```python
from build123d import *

# Parameters (mm, degrees)
F0_R            = 37.5
F1_DEPTH        = 20
F2_R            = 2
F3_DEPTH        = 20.001
F3_COPIES_COUNT = 6
F5_DEPTH        = 3.25
F5_COPIES_COUNT = 6
F6_R            = 7.5
F7_DEPTH        = 4.15
F8_W            = 7
F8_H            = 7
F9_DEPTH        = 4
F10_W           = 47
F10_H           = 3.18
F11_DEPTH       = 8.15
F12_R           = 3.25
F13_DEPTH       = 11.851


# Not quite as in the source:
# - a pattern or mirror of a feature is missing from the dataset's text; its kind, count and spacing are read off the source's solid


with BuildPart() as f1:
    # F0 (on Front) → F1 (new body)
    with BuildSketch(Plane.XZ):
        Circle(F0_R)
    extrude(amount=F1_DEPTH)

    # F2 (on Front) → F3 (cut, through all)
    with BuildSketch(Plane.XZ):
        with Locations((0, 30)):
            Circle(F2_R)
    f3 = extrude(amount=F3_DEPTH, mode=Mode.SUBTRACT)

    # F3_copies: F3 ×6 about axis
    f3_copies_axis = Axis((0, 0, 0), (0, 1, 0))
    for i in range(1, F3_COPIES_COUNT):
        add(f3.rotate(f3_copies_axis, i * 360 / F3_COPIES_COUNT), mode=Mode.SUBTRACT)

    # F4 (on face) → F5 (cut)
    with BuildSketch(Plane.XZ.offset(20)):
        Polygon((2.3749, 34.1134474629), (-2.3749, 34.1134474629), (-4.7498, 30), (-2.3749, 25.8865525371), (2.3749, 25.8865525371), (4.7498, 30), align=None)
    f5 = extrude(amount=-F5_DEPTH, mode=Mode.SUBTRACT)

    # F5_copies: F5 ×6 about axis
    f5_copies_axis = Axis((0, 0, 0), (0, 1, 0))
    for i in range(1, F5_COPIES_COUNT):
        add(f5.rotate(f5_copies_axis, i * 360 / F5_COPIES_COUNT), mode=Mode.SUBTRACT)

    # F6 (on face) → F7 (cut)
    with BuildSketch(Plane(origin=(0, 0, 0), x_dir=(-1, 0, 0), z_dir=(0, 1, 0))):
        Circle(F6_R)
    extrude(amount=-F7_DEPTH, mode=Mode.SUBTRACT)

    # F8 (on face) → F9 (cut)
    with BuildSketch(Plane(origin=(0, -4.15, 0), x_dir=(-1, 0, 0), z_dir=(0, 1, 0))):
        Rectangle(F8_W, F8_H)
    extrude(amount=-F9_DEPTH, mode=Mode.SUBTRACT)

    # F10 (on face) → F11 (cut, through all)
    with BuildSketch(Plane(origin=(0, 0, 0), x_dir=(-1, 0, 0), z_dir=(0, 1, 0))):
        Rectangle(F10_W, F10_H)
    extrude(amount=-F11_DEPTH, mode=Mode.SUBTRACT)

    # F12 (on face) → F13 (cut, through all)
    with BuildSketch(Plane(origin=(0, -8.15, 0), x_dir=(-1, 0, 0), z_dir=(0, 1, 0))):
        Circle(F12_R)
    extrude(amount=-F13_DEPTH, mode=Mode.SUBTRACT)


solid = f1.part
```
Geometry: final body of the model. Coordinates: model frame, mm. A direction names the side the tool comes from. Coordinates: 2 decimals unless noted, no trailing zeros. Loops run counter-clockwise (first coordinate to the right, second up) from the corner with the lowest first, then second, coordinate; pieces in that order, holes last. Notation, with made-up numbers: (61, 39.5) -> (80, 39.5) arc R33 cw to (80, 76.5) -> close; hole circle Ø5 at (-6, 67). An arc over 180 degrees is marked (long way). Use a Markdown table: item, result. Add a question column.
(1) Section query B-B, the plane y = -5.25. Return loops of the section in (x, z).
(2) Line query: line 1 along Z through (x, y) = (0, -12.5); line 2 along Z through (x, y) = (-26, -1); line 3 along Z through (x, y) = (21.5, -13.75). Output: solid intervals per line, ascending.
(3) Section query A-A, the plane z = 0. Return loops of the section in (x, y), plus the area to 3 significant figures.
(4) Section query C-C, the plane x = -19. Return loops of the section in (y, z), plus the area to 3 significant figures.
(5) Section query D-D, the plane y = -13. Return loops of the section in (x, z).
(6) Pin query (flat end, axial travel): pin 1 Ø1.6 at (x, y) = (0, -19) entering from -Z; pin 2 Ø2.5 at (x, z) = (0, 30) entering from -Y; pin 3 Ø0.6 at (y, z) = (-5.5, 2) entering from +X; pin 4 Ø4 at (x, y) = (-11.5, -3) entering from +Z. Return the tip coordinate at first contact, or that it passes through.
(7) Access query for faces 1 (the flat face through (-13, -4, 1.59)), 2 (the flat face through (26, -18, 19.113)), 3 (the cylindrical face through (-24.073, -8.258, -14.399)). Directions: +Z, -Z, +X, -X, +Y, -Y. A direction counts if a zero-diameter tool reaches every point of the face in a straight line with its end or side. Return the directions, or none.
Answer:
| question | item | result |
|---|---|---|
| 1 | outline | circle Ø75 at (0, 0); hole circle Ø4 at (-25.98, -15); hole circle Ø4 at (-25.98, 15); hole (-23.5, -1.59) -> (-3.5, -1.59) -> (-3.5, -3.5) -> (3.5, -3.5) -> (3.5, -1.59) -> (23.5, -1.59) -> (23.5, 1.59) -> (3.5, 1.59) -> (3.5, 3.5) -> (-3.5, 3.5) -> (-3.5, 1.59) -> (-23.5, 1.59) -> close; hole circle Ø4 at (0, -30); hole circle Ø4 at (0, 30); hole circle Ø4 at (25.98, -15); hole circle Ø4 at (25.98, 15) |
| 2 | line 1 | z = -37.5 to -32, -28 to -3.25, 3.25 to 28, 32 to 37.5 |
| 2 | line 2 | z = -27.02 to -17, -13 to 13, 17 to 27.02 |
| 2 | line 3 | z = -30.72 to 30.72 |
| 3 | outline | (-37.5, -20) -> (-3.25, -20) -> (-3.25, -8.15) -> (-23.5, -8.15) -> (-23.5, 0) -> (-37.5, 0) -> close; (3.25, -20) -> (37.5, -20) -> (37.5, 0) -> (23.5, 0) -> (23.5, -8.15) -> (3.25, -8.15) -> close |
| 3 | area | 1,040 mm^2 |
| 4 | outline | (-20, -32.33) -> (0, -32.33) -> (0, -1.59) -> (-8.15, -1.59) -> (-8.15, 1.59) -> (0, 1.59) -> (0, 32.33) -> (-20, 32.33) -> close |
| 4 | area | 1,270 mm^2 |
| 5 | outline | circle Ø75 at (0, 0); hole circle Ø4 at (-25.98, -15); hole circle Ø4 at (-25.98, 15); hole circle Ø6.5 at (0, 0); hole circle Ø4 at (0, -30); hole circle Ø4 at (0, 30); hole circle Ø4 at (25.98, -15); hole circle Ø4 at (25.98, 15) |
| 6 | pin 1 | stops at z = -37.5 |
| 6 | pin 2 | passes through |
| 6 | pin 3 | stops at x = 37.46 |
| 6 | pin 4 | stops at z = 36.28 |
| 7 | face 1 | +Y |
| 7 | face 2 | -Y |
| 7 | face 3 | +Y, -Y |
